from build123d import *

# Parameters (mm, degrees)
CROQUIS1_W                   = 75
CROQUIS1_H                   = 35
CROQUIS1_R                   = 2.25
SALIENTE_EXTRUIR1_DEPTH      = 3
TALADRO_DE_MARGEN_PARA_M41_D = 4.5
TALADRO_DE_MARGEN_PARA_M21_D = 2.4
CROQUIS6_W                   = 15
CROQUIS6_H                   = 6
SALIENTE_EXTRUIR2_DEPTH      = 6
REDONDEO1_SIZE               = 8


with BuildPart() as part:
    # Croquis1 → Saliente-Extruir1 (new, symmetric)
    with BuildSketch(Plane.XY):
        Rectangle(CROQUIS1_W, CROQUIS1_H)
        with Locations((-11.25, 5)):
            Circle(CROQUIS1_R, mode=Mode.SUBTRACT)
        with BuildLine():
            ThreePointArc((14.62076493, -0.557692308), (11.25, 11.5), (7.87923507, -0.557692308))
            ThreePointArc((7.87923507, -0.557692308), (11.25, -5), (14.62076493, -0.557692308))
        make_face(mode=Mode.SUBTRACT)
    extrude(amount=SALIENTE_EXTRUIR1_DEPTH, both=True)

    # Taladro de margen para M41 (through all)
    with Locations(Plane.XY.offset(3)):
        with Locations((-31.25, 5), (31.25, 5), (21.25, -10), (-21.25, -10)):
            Hole(TALADRO_DE_MARGEN_PARA_M41_D / 2)

    # Taladro de margen para M21 (through all)
    with Locations(Plane.XY.offset(3)):
        with Locations((11.25, 13.35), (11.25, -13.85)):
            Hole(TALADRO_DE_MARGEN_PARA_M21_D / 2)

    # Croquis6 → Saliente-Extruir2 (add, through all)
    with BuildSketch(Plane.XY.offset(3)):
        with Locations((-17.5, -20.5)):
            Rectangle(CROQUIS6_W, CROQUIS6_H)
        with Locations((17.5, -20.5)):
            Rectangle(CROQUIS6_W, CROQUIS6_H)
    extrude(amount=-SALIENTE_EXTRUIR2_DEPTH)

    # Redondeo1
    redondeo1_edges = [part.edges().sort_by_distance(p)[0] for p in [
        (-37.5, 17.5, 0),
        (37.5, 17.5, 0),
        (37.5, -17.5, 0),
        (-37.5, -17.5, 0),
    ]]
    chamfer(redondeo1_edges, length=REDONDEO1_SIZE)


solid = part.part
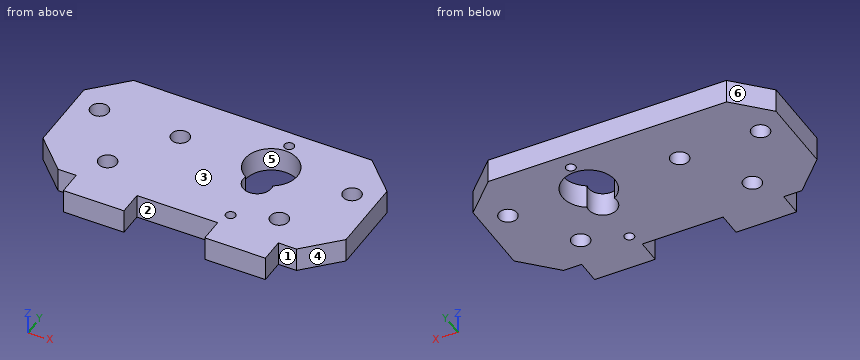
Could you check a few things on this model? Use its own coordinates, in mm. Face numbers are marked on the shaded views. A direction names the side the tool comes from. Give positions to 0.01 mm unless a question says otherwise; leave off trailing zeros. Order: outer loops, then holes, each group sorted by start corner. A loop starts at its lowest first (then second) coordinate and runs counter-clockwise, first axis right, second up.
1. Suppose I cut it at C-C (y = 13.35). List the corners of the cut face in (x, z) for me.
2. Suppose I cut it at B-B (y = 5). List the corners of the cut face in (x, z) for me.
3. I need wall thicknesses on L1, parallel to X at y = 5.5, z = 1; L2, parallel to X at y = -9, z = 2.75; L3, parallel to X at y = 3, z = 1.25. Which ranges of each line are inside material? Lowest first, please.
4. Will these pins go through, and if not, where does the flat tip stop? P1, Ø3, axis at y = -22, z = 1, coming from the -X side; P2, Ø6, axis at x = -31.25, y = 5, coming from the -Z side; P3, Ø1.3, axis at x = 28, z = 0, coming from the -Y side.
5. For the marked faces 1, 2 and 3, which set-ups out of +Z, -Z, +X, -X, +Y, -Y let a thin tool reach every point of the face, with its end or its side?
6. Suppose I cut it at D-D (x = 11.25). List the corners of the cut face in (y, z) for me, plus the area to 3 significant figures.
7. Suppose I cut it at A-A (x = -11.25). List the corners of the cut face in (y, z) for me, plus the area to 3 significant figures.
8. We'd pull the mould along Y, two halves only. Please class the marked faces 4, 5 and 6: pulls with the +Y half, pulls with the -Y half, needs draft (parallel to the pull), parting line crosses it, or undercut.
Solved:
1. outline: (-33.65, -3) - (10.05, -3) - (10.05, 3) - (-33.65, 3) - close; (12.45, -3) - (33.65, -3) - (33.65, 3) - (12.45, 3) - close
2. outline: (-37.5, -3) - (-33.5, -3) - (-33.5, 3) - (-37.5, 3) - close; (-29, -3) - (-13.5, -3) - (-13.5, 3) - (-29, 3) - close; (-9, -3) - (4.75, -3) - (4.75, 3) - (-9, 3) - close; (17.75, -3) - (29, -3) - (29, 3) - (17.75, 3) - close; (33.5, -3) - (37.5, -3) - (37.5, 3) - (33.5, 3) - close
3. L1: x = -37.5 to -33.44, -29.06 to -13.44, -9.06 to 4.77, 17.73 to 29.06, 33.44 to 37.5
3. L2: x = -37.5 to -23.27, -19.23 to 19.23, 23.27 to 37.5
3. L3: x = -37.5 to -32.28, -30.22 to -12.28, -10.22 to 5.07, 17.43 to 30.22, 32.28 to 37.5
4. P1: stops at x = -25
4. P2: stops at z = -3
4. P3: stops at y = -17.5
5. face 1: +Z, -Z, +X, -Y
5. face 2: +Z, -Z, -Y
5. face 3: +Z, +X, -X, +Y, -Y
6. outline: (-23.5, -3) - (-15.05, -3) - (-15.05, 3) - (-23.5, 3) - close; (-12.65, -3) - (-5, -3) - (-5, 3) - (-12.65, 3) - close; (11.5, -3) - (12.15, -3) - (12.15, 3) - (11.5, 3) - close; (14.55, -3) - (17.5, -3) - (17.5, 3) - (14.55, 3) - close
6. area: 118 mm2
7. outline: (-23.5, -3) - (2.75, -3) - (2.75, 3) - (-23.5, 3) - close; (7.25, -3) - (17.5, -3) - (17.5, 3) - (7.25, 3) - close
7. area: 219 mm2
8. face 4: pulls with the -Y half
8. face 5: undercut
8. face 6: pulls with the +Y half
